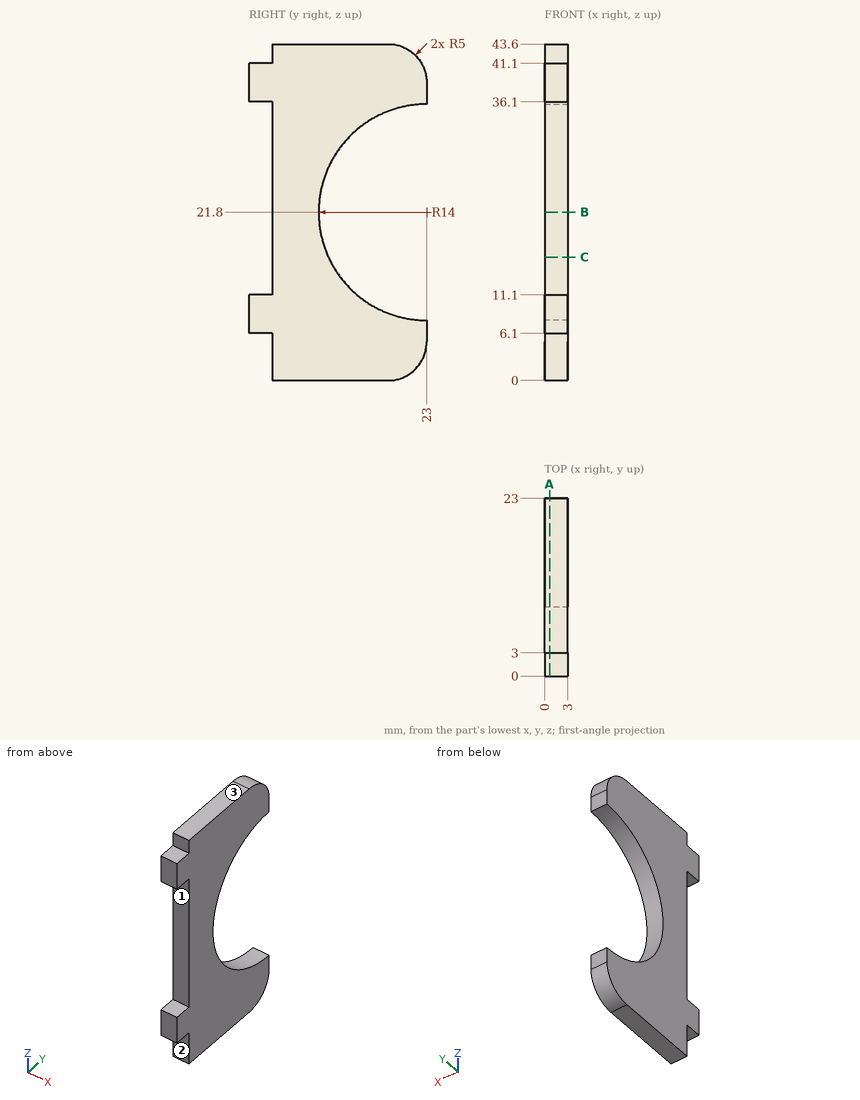
The figure shows three views and two pictorial views of one solid part (mm, origin at its lowest corner). Answer the questions. Coordinates: 2 decimals unless noted, no trailing zeros. Loops run counter-clockwise (first coordinate to the right, second up) from the corner with the lowest first, then second, coordinate; pieces in that order, holes last. Notation, with made-up numbers: (-29, 87.25) - (10, 87.25) arc R14 cw to (10, 103.25) - close; hole circle Ø10 at (-6, 38.5). An arc over 180 degrees is marked (long way). Use a Markdown table: item, result. Add a question column.
1) Find the intervals of material crossed by line 1 (Z direction, x = 1.7, y = 20); line 2 (Z direction, x = 2.5, y = 15); line 3 (Y direction, x = 0.5, z = 22), in increasing order.
2) The part is cut by section B-B, the plane z = 21.8. Give the vertices of the cut face in (x, y), and give its area (3 significant figures).
3) The part is cut by section A-A, the plane x = 0.65. Give the vertices of the cut face in (y, z), and give its area (3 significant figures).
4) Given pin 1 (0.9 mm diameter, centred on x = 1, y = 2, fed in from +Z), flat-ended and moving along its own axis, determine where the tip first touches the part or whether it passes through.
5) The mould has two halves that part along Z. Classify the marked faces 1, 2 and 3: released by +Z, released by -Z, zero draft, split by the parting line, or undercut.
6) The part is cut by section C-C, the plane z = 16. Give the vertices of the cut face in (x, y).
Here are the results:
| question | item | result |
|---|---|---|
| 1 | line 1 | z = 0.42 to 8.13, 35.47 to 43.18 |
| 1 | line 2 | z = 0 to 10.31, 33.29 to 43.6 |
| 1 | line 3 | y = 3 to 9 |
| 2 | outline | (0, 3) - (3, 3) - (3, 9) - (0, 9) - close |
| 2 | area | 18.0 mm^2 |
| 3 | outline | (0, 6.1) - (3, 6.1) - (3, 0) - (18, 0) arc R5 ccw to (23, 5) - (23, 7.8) arc R14 cw to (23, 35.8) - (23, 38.6) arc R5 ccw to (18, 43.6) - (3, 43.6) - (3, 41.1) - (0, 41.1) - (0, 36.1) - (3, 36.1) - (3, 11.1) - (0, 11.1) - close |
| 3 | area | 583 mm^2 |
| 4 | pin 1 | stops at z = 41.1 |
| 5 | face 1 | undercut |
| 5 | face 2 | zero draft |
| 5 | face 3 | released by +Z |
| 6 | outline | (0, 3) - (3, 3) - (3, 10.26) - (0, 10.26) - close |
